from build123d import *

# Parameters (mm, degrees)
F0_R          = 24.4
F0_R_2        = 18.36585117
F1_DEPTH      = 60
F2_R          = 24.4
F2_R_2        = 18.36585117
F3_DEPTH      = 1425
F4_R          = 7.5
F5_DEPTH      = 24.401
F5_DEPTH_BACK = 24.401


with BuildPart() as f1:
    # F0 (on Top) → F1 (new body)
    with BuildSketch(Plane.XY):
        Circle(F0_R)
        Circle(F0_R_2, mode=Mode.SUBTRACT)
    extrude(amount=F1_DEPTH)

    # F2 (on Top) → F3 (join)
    with BuildSketch(Plane.XY):
        Circle(F2_R)
        Circle(F2_R_2, mode=Mode.SUBTRACT)
    extrude(amount=-F3_DEPTH)

    # F4 (on Front) → F5 (cut, two sides)
    with BuildSketch(Plane.XZ) as f5_sk:
        with Locations((0, 37.5)):
            Circle(F4_R)
    extrude(amount=-F5_DEPTH, mode=Mode.SUBTRACT)
    extrude(f5_sk.sketch, amount=F5_DEPTH_BACK, mode=Mode.SUBTRACT)


solid = f1.part
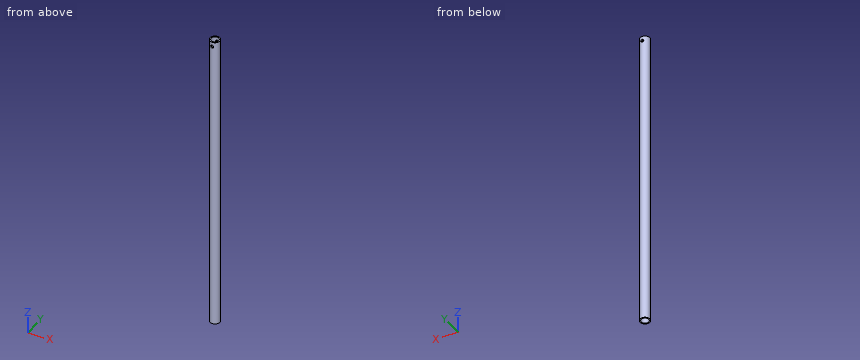
Model file for the job. Use its own axes, mm. Give positions to 0.01 mm unless a question says otherwise; leave off trailing zeros. Order: outer loops, then holes, each group sorted by start corner. A loop starts at its lowest first (then second) coordinate and runs counter-clockwise, first axis right, second up. Notation, with made-up numbers: (9, 69) - (46, 69) arc R22 cw to (46, 95) - close; hole circle Ø4 at (58, 89). An arc over 180 degrees is marked (long way). Write item = value, one per line. Start each with the question number.
1. Drop flat-ended pins along their axis: P1, Ø10, axis at x = 3.5, y = 12.5, coming from the -Z side; P2, Ø2, axis at x = -7, z = -188.5, coming from the +Y side; P3, Ø2, axis at y = 19, z = -862.5, coming from the -X side; P4, Ø10, axis at y = -11, z = -797, coming from the -X side. Give the stop position or say it passes through.
2. Cut at B-B, the plane z = -411.5. List the corners of the cut face in (x, y), and give its area (3 significant figures).
3. Cut at A-A, the plane y = 0. List the corners of the cut face in (x, z).
4. Probe line 1 along Y through (x, z) = (-2, -930.5); line 2 along X through (y, z) = (-0.5, -362.5); line 3 along Z through (x, y) = (0, -19.25). List the from-to ranges inside material, lowest first.
Taken from the geometry:
q1.P1 = through
q1.P2 = 23.65
q1.P3 = -16.47
q1.P4 = -23.65
q2.outline = circle Ø48.8 at (0, 0); hole circle Ø36.73 at (0, 0)
q2.area = 811 mm²
q3.outline = (-24.4, -1425) - (-18.37, -1425) - (-18.37, 60) - (-24.4, 60) - close; (18.37, -1425) - (24.4, -1425) - (24.4, 60) - (18.37, 60) - close
q4.line_1 = -24.32 to -18.26, 18.26 to 24.32
q4.line_2 = -24.39 to -18.36, 18.36 to 24.39
q4.line_3 = -1425 to 30, 45 to 60
